Geometry check sheet. Reference: drawing and pictorial views, mm from the part's lowest x, y, z. Coordinates: 2 decimals unless noted, no trailing zeros. Loops run counter-clockwise (first coordinate to the right, second up) from the corner with the lowest first, then second, coordinate; pieces in that order, holes last. Notation, with made-up numbers: (-34.5, 49) -> (-0.5, 49) arc R38 ccw to (-0.5, 88) -> close; hole circle Ø9 at (64.25, 56.25). An arc over 180 degrees is marked (long way). Answer as a JSON object with one key per item and string values. Group by question number.
Q1. Cross-section at B-B on x = 7.5. Record the boundary of the cut face in (y, z).
Q2. Cross-section at C-C on x = 79. Record the boundary of the cut face in (y, z).
Q3. Cross-section at A-A on z = 15. Record the boundary of the cut face in (x, y).
Q4. Scan lines: L1, parallel to Y at x = 91.5, z = 22.5; L2, parallel to Z at x = 65, y = 27; L3, parallel to Z at x = 19, y = 14. Record each from-to range of solid material in increasing order.
Q5. Gauge pin test, flat ends, axial feed: pin 1 Ø1.5 at (x, z) = (71.5, 16) entering from -Y; pin 2 Ø6.5 at (x, z) = (78, 14.5) entering from +Y; pin 3 Ø3 at (x, y) = (81.5, 27.5) entering from +Z. Record the tip position at first contact, or that the pin passes through.
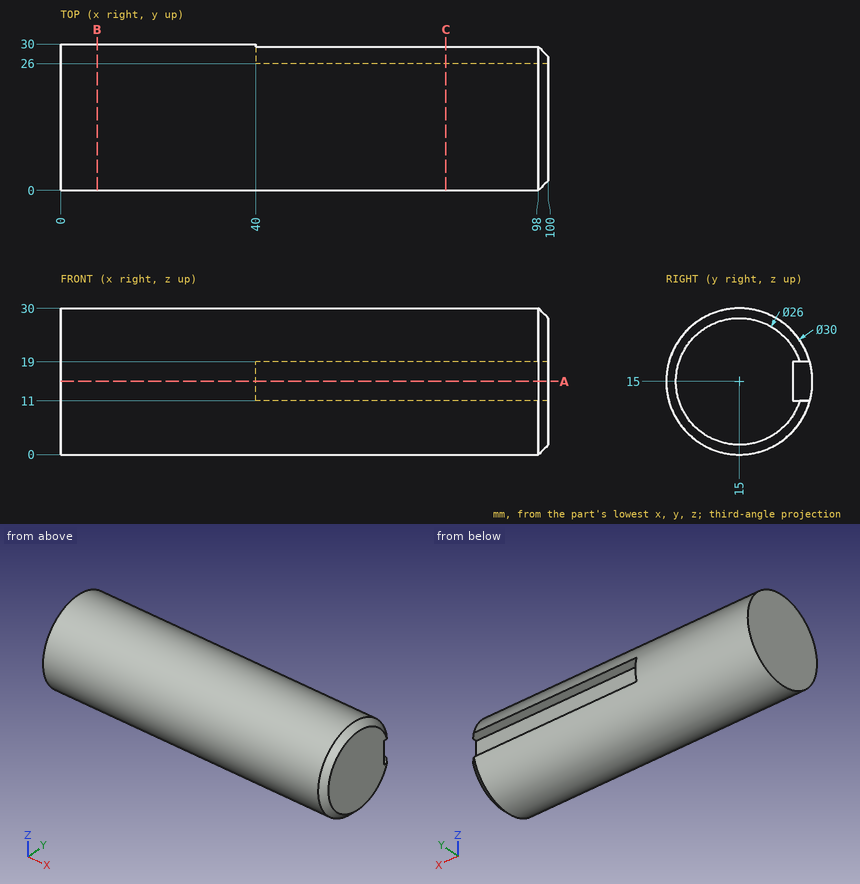
Computed values:
{
 "1": {"outline": "circle Ø30 at (15, 15)"},
 "2": {"outline": "(26, 11) -> (26, 19) -> (29.46, 19) arc R15 ccw (long way) to (29.46, 11) -> close"},
 "3": {"outline": "(0, 0) -> (98, 0) -> (100, 2) -> (100, 26) -> (40, 26) -> (40, 30) -> (0, 30) -> close"},
 "4": {"L1": "y = 2.01 to 27.99", "L2": "z = 6 to 11, 19 to 24", "L3": "z = 0.03 to 29.97"},
 "5": {"pin 1": "stops at y = 0", "pin 2": "stops at y = 26", "pin 3": "stops at z = 25.2"}
}
